Geometry check sheet. Reference: the model listing, model coordinates, mm. A direction names the side the tool comes from. Give positions to 0.01 mm unless a question says otherwise; leave off trailing zeros. Write each loop counter-clockwise with the first axis right and the second up, starting at its lowest first coordinate (ties: lowest second). Pieces come first, ordered by that corner, then holes. Notation, with made-up numbers: (64, -31.5) - (75, -31.5) arc R23 cw to (75, -17.5) - close; hole circle Ø9 at (-21.75, 22). An arc over 180 degrees is marked (long way). Write item = value, one per line. Start each with the question number.
(1) Depth check by flat-ended pin: pin 1 Ø3 at (x, z) = (-9, -5) entering from +Y; pin 2 Ø1 at (x, y) = (2.5, 8.5) entering from +Z; pin 3 Ø1.2 at (x, y) = (-6.5, 5.5) entering from -Z; pin 4 Ø2.5 at (x, z) = (-9.5, -5) entering from -Y. Enter the tip coordinate at first touch or a pass-through.
(2) Access from +Z, -Z, +X, -X, +Y, -Y to the whole of each face (thin tool, end or side, straight path). Record for faces 1 (the flat face through (0.5, 2, 0)), 2 (the flat face through (1.16, 9.028, 9.677)), 3 (the cylindrical face through (15.141, 5.028, 11.143)).
(3) Draft check along Z on faces 4 (the conical face through (15.065, 9.028, -10.979)), 5 (the flat face through (-4, 11, 10)), 6 (the flat face through (1, 5, 9.5)). Enter one of: pulls with the +Z half, pulls with the -Z half, needs draft (parallel to the pull), parting line crosses it, or undercut.
(4) Section check B-B, the plane z = -5. Enter the section's corners in (x, y), plus the area to 3 significant figures.
(5) Section check A-A, the plane y = 2. Enter the section's corners in (x, z).
(6) Thickness scan on L1, parallel to X at y = 1.9, z = 5; L2, parallel to Z at x = -3.5, y = 6.25; L3, parallel to Z at x = -5, y = 2.5. Record the ranges inside material, lowest first.
(7) Section check D-D, the plane z = 1. Enter the section's corners in (x, y), plus the area to 3 significant figures.
(8) Section check C-C, the plane x = 3.5. Enter the section's corners in (y, z), plus the area to 3 significant figures.
```python
from build123d import *
from OCP.BRepFilletAPI import BRepFilletAPI_MakeChamfer

# Parameters (mm, degrees)
SKETCH1_W           = 36
SKETCH1_H           = 27
BOSS_EXTRUDE1_DEPTH = 3
SKETCH2_W           = 6
SKETCH2_H           = 6
CUT_EXTRUDE1_DEPTH  = 1.5
SKETCH3_R           = 1.45
CUT_EXTRUDE2_DEPTH  = 2.3
BOSS_EXTRUDE3_DEPTH = 8
FILLET1_R           = 2
FILLET2_R           = 0.5
FILLET3_R           = 0.5
CHAMFER2_SIZE       = 4
CHAMFER2_SIZE2      = 0.349954654


with BuildPart() as part:
    # Sketch1 → Boss-Extrude1 (new body)
    with BuildSketch(Plane(origin=(0, 0, 0), x_dir=(1, 0, 0), z_dir=(0, 1, 0))):
        Rectangle(SKETCH1_W, SKETCH1_H)
    extrude(amount=BOSS_EXTRUDE1_DEPTH)

    # Sketch2 → Cut-Extrude1 (cut)
    with BuildSketch(Plane(origin=(0, 3, 0), x_dir=(1, 0, 0), z_dir=(0, 1, 0))):
        with Locations((-2.5, 0)):
            Rectangle(SKETCH2_W, SKETCH2_H)
    extrude(amount=-CUT_EXTRUDE1_DEPTH, mode=Mode.SUBTRACT)

    # Sketch3 → Cut-Extrude2 (cut)
    with BuildSketch(Plane(origin=(0, 3, 0), x_dir=(1, 0, 0), z_dir=(0, 1, 0))):
        with Locations(Location((-9.5, 5, 0), (0, 0, 270))):
            Circle(SKETCH3_R)
        with Locations(Location((-9.5, -5, 0), (0, 0, 90))):
            Circle(SKETCH3_R)
    extrude(amount=-CUT_EXTRUDE2_DEPTH, mode=Mode.SUBTRACT)

    # Sketch4 → Boss-Extrude3 (add)
    with BuildSketch(Plane(origin=(0, 3, 0), x_dir=(1, 0, 0), z_dir=(0, 1, 0))):
        Polygon((-16, 11.5), (-16, -11.5), (16, -11.5), (16, -9.5), (-14, -9.5), (-14, 9.5), (16, 9.5), (16, 11.5), align=None)
    extrude(amount=BOSS_EXTRUDE3_DEPTH)

    # Fillet1
    fillet1_edges = [part.edges().sort_by_distance(p)[0] for p in [
        (-16, 7, -11.5),
        (16, 7, -11.5),
        (16, 7, 11.5),
        (-16, 7, 11.5),
        (-18, 1.5, 13.5),
        (18, 1.5, 13.5),
        (-18, 1.5, -13.5),
        (18, 1.5, -13.5),
    ]]
    fillet(fillet1_edges, radius=FILLET1_R - 0.0001)  # a hair under: the kernel refuses the full size

    # Fillet2
    fillet2_edges = [part.edges().sort_by_distance(p)[0] for p in [
        (-14, 7, 9.5),
        (-14, 7, -9.5),
    ]]
    fillet(fillet2_edges, radius=FILLET2_R)

    # Fillet3
    fillet3_edges = [part.edges().sort_by_distance(p)[0] for p in [
        (0.5, 2.25, -3),
        (0.5, 2.25, 3),
        (-5.5, 2.25, 3),
        (-5.5, 2.25, -3),
        (16, 7, 9.5),
        (16, 7, -9.5),
    ]]
    fillet(fillet3_edges, radius=FILLET3_R)

    # Chamfer2: one chamfer whose edges measure the first distance from different faces: ONE call of the kernel's chamfer builder (chamfer() names one face for all edges)
    chamfer2_edges_1 = [part.edges().sort_by_distance(p)[0] for p in [
        (0.957121425, 11, -9.5),
    ]]
    chamfer2_side_1 = [part.faces().sort_by_distance(p)[0] for p in [
        (0.957121425, 7, -9.5),
    ]]
    chamfer2_edges_2 = [part.edges().sort_by_distance(p)[0] for p in [
        (-14, 11, 0),
    ]]
    chamfer2_side_2 = [part.faces().sort_by_distance(p)[0] for p in [
        (-14, 7, 0),
    ]]
    chamfer2_edges_3 = [part.edges().sort_by_distance(p)[0] for p in [
        (-13.853553391, 11, -9.353553391),
    ]]
    chamfer2_side_3 = [part.faces().sort_by_distance(p)[0] for p in [
        (-13.853553391, 7, -9.353553391),
    ]]
    chamfer2_edges_4 = [part.edges().sort_by_distance(p)[0] for p in [
        (-13.853553391, 11, 9.353553391),
    ]]
    chamfer2_side_4 = [part.faces().sort_by_distance(p)[0] for p in [
        (-13.853553391, 7, 9.353553391),
    ]]
    chamfer2_edges_5 = [part.edges().sort_by_distance(p)[0] for p in [
        (15.154781293, 11, -11.132984295),
    ]]
    chamfer2_side_5 = [part.faces().sort_by_distance(p)[0] for p in [
        (15.154781293, 7, -11.132984295),
    ]]
    chamfer2_edges_6 = [part.edges().sort_by_distance(p)[0] for p in [
        (0.957121425, 11, 9.5),
    ]]
    chamfer2_side_6 = [part.faces().sort_by_distance(p)[0] for p in [
        (0.957121425, 7, 9.5),
    ]]
    chamfer2_edges_7 = [part.edges().sort_by_distance(p)[0] for p in [
        (15.822484336, 11, 9.711315242),
    ]]
    chamfer2_side_7 = [part.faces().sort_by_distance(p)[0] for p in [
        (15.822484336, 7, 9.711315242),
    ]]
    chamfer2_edges_8 = [part.edges().sort_by_distance(p)[0] for p in [
        (15.822484336, 11, -9.711315242),
    ]]
    chamfer2_side_8 = [part.faces().sort_by_distance(p)[0] for p in [
        (15.822484336, 7, -9.711315242),
    ]]
    chamfer2_edges_9 = [part.edges().sort_by_distance(p)[0] for p in [
        (-16, 11, 0),
    ]]
    chamfer2_side_9 = [part.faces().sort_by_distance(p)[0] for p in [
        (-16, 7, 0),
    ]]
    chamfer2_edges_10 = [part.edges().sort_by_distance(p)[0] for p in [
        (0, 11, -11.5),
    ]]
    chamfer2_side_10 = [part.faces().sort_by_distance(p)[0] for p in [
        (0, 7, -11.5),
    ]]
    chamfer2_edges_11 = [part.edges().sort_by_distance(p)[0] for p in [
        (0, 11, 11.5),
    ]]
    chamfer2_side_11 = [part.faces().sort_by_distance(p)[0] for p in [
        (0, 7, 11.5),
    ]]
    chamfer2_edges_12 = [part.edges().sort_by_distance(p)[0] for p in [
        (-15.414242852, 11, 10.914242852),
    ]]
    chamfer2_side_12 = [part.faces().sort_by_distance(p)[0] for p in [
        (-15.414242852, 7, 10.914242852),
    ]]
    chamfer2_edges_13 = [part.edges().sort_by_distance(p)[0] for p in [
        (15.154781293, 11, 11.132984295),
    ]]
    chamfer2_side_13 = [part.faces().sort_by_distance(p)[0] for p in [
        (15.154781293, 7, 11.132984295),
    ]]
    chamfer2_edges_14 = [part.edges().sort_by_distance(p)[0] for p in [
        (-15.414242852, 11, -10.914242852),
    ]]
    chamfer2_side_14 = [part.faces().sort_by_distance(p)[0] for p in [
        (-15.414242852, 7, -10.914242852),
    ]]
    chamfer2 = BRepFilletAPI_MakeChamfer(part.part.solid().wrapped)
    for e in chamfer2_edges_1:
        chamfer2.Add(CHAMFER2_SIZE, CHAMFER2_SIZE2, e.wrapped, chamfer2_side_1[0].wrapped)  # the first distance lies on this face
    for e in chamfer2_edges_2:
        chamfer2.Add(CHAMFER2_SIZE, CHAMFER2_SIZE2, e.wrapped, chamfer2_side_2[0].wrapped)  # the first distance lies on this face
    for e in chamfer2_edges_3:
        chamfer2.Add(CHAMFER2_SIZE, CHAMFER2_SIZE2, e.wrapped, chamfer2_side_3[0].wrapped)  # the first distance lies on this face
    for e in chamfer2_edges_4:
        chamfer2.Add(CHAMFER2_SIZE, CHAMFER2_SIZE2, e.wrapped, chamfer2_side_4[0].wrapped)  # the first distance lies on this face
    for e in chamfer2_edges_5:
        chamfer2.Add(CHAMFER2_SIZE, CHAMFER2_SIZE2, e.wrapped, chamfer2_side_5[0].wrapped)  # the first distance lies on this face
    for e in chamfer2_edges_6:
        chamfer2.Add(CHAMFER2_SIZE, CHAMFER2_SIZE2, e.wrapped, chamfer2_side_6[0].wrapped)  # the first distance lies on this face
    for e in chamfer2_edges_7:
        chamfer2.Add(CHAMFER2_SIZE, CHAMFER2_SIZE2, e.wrapped, chamfer2_side_7[0].wrapped)  # the first distance lies on this face
    for e in chamfer2_edges_8:
        chamfer2.Add(CHAMFER2_SIZE, CHAMFER2_SIZE2, e.wrapped, chamfer2_side_8[0].wrapped)  # the first distance lies on this face
    for e in chamfer2_edges_9:
        chamfer2.Add(CHAMFER2_SIZE, CHAMFER2_SIZE2, e.wrapped, chamfer2_side_9[0].wrapped)  # the first distance lies on this face
    for e in chamfer2_edges_10:
        chamfer2.Add(CHAMFER2_SIZE, CHAMFER2_SIZE2, e.wrapped, chamfer2_side_10[0].wrapped)  # the first distance lies on this face
    for e in chamfer2_edges_11:
        chamfer2.Add(CHAMFER2_SIZE, CHAMFER2_SIZE2, e.wrapped, chamfer2_side_11[0].wrapped)  # the first distance lies on this face
    for e in chamfer2_edges_12:
        chamfer2.Add(CHAMFER2_SIZE, CHAMFER2_SIZE2, e.wrapped, chamfer2_side_12[0].wrapped)  # the first distance lies on this face
    for e in chamfer2_edges_13:
        chamfer2.Add(CHAMFER2_SIZE, CHAMFER2_SIZE2, e.wrapped, chamfer2_side_13[0].wrapped)  # the first distance lies on this face
    for e in chamfer2_edges_14:
        chamfer2.Add(CHAMFER2_SIZE, CHAMFER2_SIZE2, e.wrapped, chamfer2_side_14[0].wrapped)  # the first distance lies on this face
    add(Compound.cast(chamfer2.Shape()), mode=Mode.REPLACE)


solid = part.part
```
Model answer:
q1.pin_1 = 3
q1.pin_2 = 11.41
q1.pin_3 = -11.5
q1.pin_4 = 0
q2.face_1 = +Y
q2.face_2 = +X, +Y
q2.face_3 = +Z, +X, +Y
q3.face_4 = pulls with the -Z half
q3.face_5 = needs draft
q3.face_6 = undercut
q4.outline = (-18, 0) - (18, 0) - (18, 3) - (-8.05, 3) - (-8.05, 0.7) - (-10.95, 0.7) - (-10.95, 3) - (-14, 3) - (-14, 7) - (-14.35, 11) - (-15.65, 11) - (-16, 7) - (-16, 3) - (-18, 3) - close
q4.area = 116 mm²
q5.outline = (-18, -11.5) arc R2 ccw to (-16, -13.5) - (16, -13.5) arc R2 ccw to (18, -11.5) - (18, 11.5) arc R2 ccw to (16, 13.5) - (-16, 13.5) arc R2 ccw to (-18, 11.5) - close; hole circle Ø2.9 at (-9.5, -5); hole circle Ø2.9 at (-9.5, 5); hole (-5.5, -2.5) arc R0.5 ccw to (-5, -3) - (0, -3) arc R0.5 ccw to (0.5, -2.5) - (0.5, 2.5) arc R0.5 ccw to (0, 3) - (-5, 3) arc R0.5 ccw to (-5.5, 2.5) - close
q6.L1 = -18 to -10.95, -8.05 to 18
q6.L2 = -11.5 to -9.5, 9.5 to 11.5
q6.L3 = -13.5 to -3, 3 to 13.5
q7.outline = (-18, 0) - (18, 0) - (18, 3) - (0.5, 3) - (0.5, 1.5) - (-5.5, 1.5) - (-5.5, 3) - (-14, 3) - (-14, 7) - (-14.35, 11) - (-15.65, 11) - (-16, 7) - (-16, 3) - (-18, 3) - close
q7.area = 114 mm²
q8.outline = (0, -13.5) - (3, -13.5) - (3, -11.5) - (7, -11.5) - (11, -11.15) - (11, -9.85) - (7, -9.5) - (3, -9.5) - (3, 9.5) - (7, 9.5) - (11, 9.85) - (11, 11.15) - (7, 11.5) - (3, 11.5) - (3, 13.5) - (0, 13.5) - close
q8.area = 110 mm²
